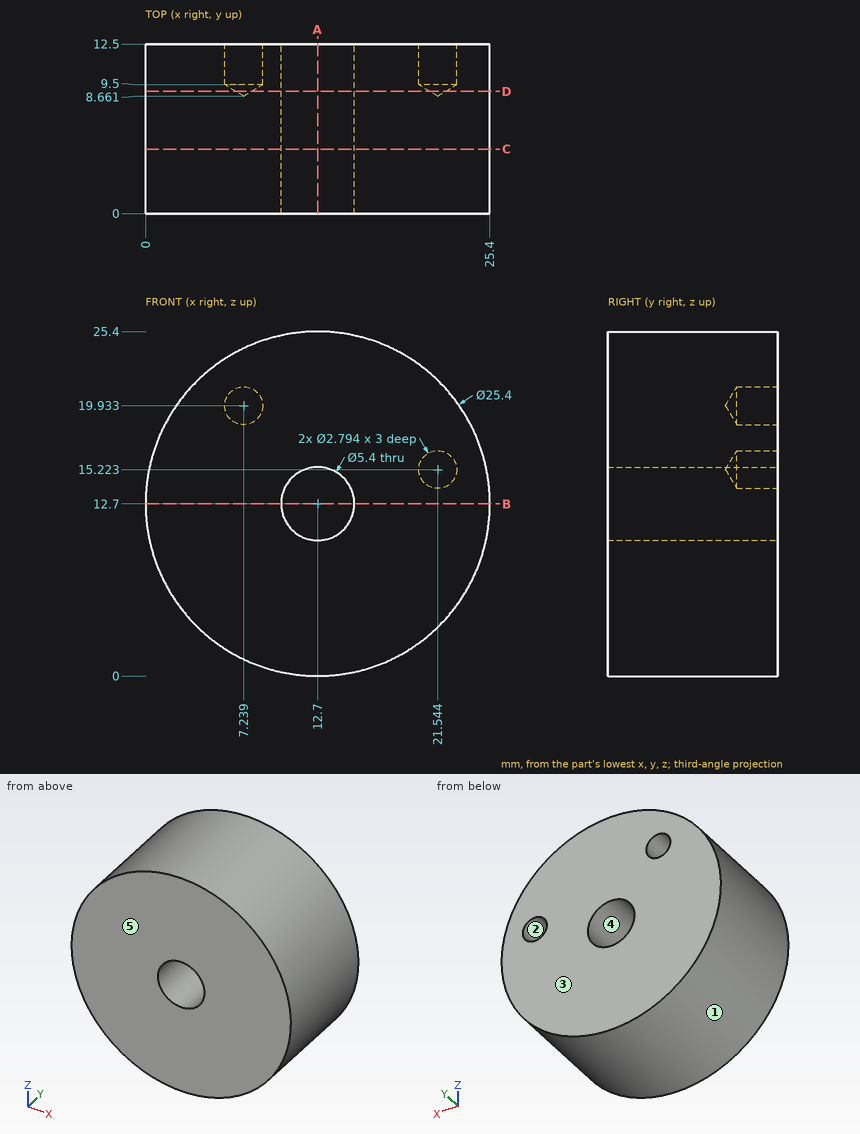
Part print with two shaded views. Sizes in mm from the minimum x, y, z corner. A direction names the side the tool comes from. Coordinates: 2 decimals unless noted, no trailing zeros. Order: outer loops, then holes, each group sorted by start corner. A loop starts at its lowest first (then second) coordinate and runs counter-clockwise, first axis right, second up. Notation, with made-up numbers: (73.5, -22) - (96.5, -22) arc R19 ccw to (96.5, -11) - close; hole circle Ø8 at (76, 52). An arc over 180 degrees is marked (long way). Answer in a Markdown table with one row per item.
1. Pull direction Y, two halves, no side cores. Call the marked faces 3, 4 and 5: +Y half, -Y half, draft (parallel to the pull), parting line (faces both ways), or undercut.
Answer:
| item | result |
|---|---|
| face 3 | +Y half |
| face 4 | draft |
| face 5 | -Y half |
2. Flat gauge pins, fed straight in: P1, Ø2, axis at y = 11, z = 7.5, coming from the -X side (1 decimal); P2, Ø1.5, axis at y = 7, z = 18.5, coming from the +X side; P3, Ø2, axis at x = 15, y = 5, coming from the +Z side. Where does each tip first touch, or does it go through?
Answer:
| item | result |
|---|---|
| P1 | x = 0.7 |
| P2 | x = 24.35 |
| P3 | z = 25.33 |
3. Slice it at D-D, the plane y = 9. List the corners of the cut face in (x, z) (1 decimal), then the cut area to 3 significant figures.
Answer:
| item | result |
|---|---|
| outline | circle Ø25.4 at (12.7, 12.7); hole circle Ø1.1 at (7.2, 19.9); hole circle Ø5.4 at (12.7, 12.7); hole circle Ø1.1 at (21.5, 15.2) |
| area | 482 mm² |
4. Slice it at B-B, the plane z = 12.7. List the corners of the cut face in (x, y).
Answer:
| item | result |
|---|---|
| outline | (0, 0) - (10, 0) - (10, 12.5) - (0, 12.5) - close; (15.4, 0) - (25.4, 0) - (25.4, 12.5) - (15.4, 12.5) - close |
5. Slice it at A-A, the plane x = 12.7. List the corners of the cut face in (y, z).
Answer:
| item | result |
|---|---|
| outline | (0, 0) - (12.5, 0) - (12.5, 10) - (0, 10) - close; (0, 15.4) - (12.5, 15.4) - (12.5, 25.4) - (0, 25.4) - close |
6. Slice it at C-C, the plane y = 4.75. List the corners of the cut face in (x, z).
Answer:
| item | result |
|---|---|
| outline | circle Ø25.4 at (12.7, 12.7); hole circle Ø5.4 at (12.7, 12.7) |
7. 3-axis set-ups, long thin cutter, end or side, ignore diameter. For the marked faces 1 and 2: which of +Z, -Z, +X, -X, +Y, -Y reach the whole face in a straight line?
Answer:
| item | result |
|---|---|
| face 1 | +Y, -Y |
| face 2 | +Y |
8. Drill centre lines: L1, parallel to Z at x = 12.75, y = 10.75; L2, parallel to Z at x = 21, y = 10.5 (1 decimal). Where is each one in solid material? Low to high. Write a range as from..to.
Answer:
| item | result |
|---|---|
| L1 | 0..10, 15.4..25.4 |
| L2 | 3.1..13.9, 16.5..22.3 |
